Geometry check sheet. Reference: the model listing, model coordinates, mm. A direction names the side the tool comes from. Give positions to 0.01 mm unless a question says otherwise; leave off trailing zeros. Write each loop counter-clockwise with the first axis right and the second up, starting at its lowest first coordinate (ties: lowest second). Pieces come first, ordered by that corner, then holes. Notation, with made-up numbers: M 59,-38.75 L 94,-38.75 A14 cw 94,-19.75 Z; hole C -27,54 d4. An arc over 180 degrees is marked long. One line per item, written item: value. Start each with the question number.
1. Cross-section at C-C on y = 15. Record the cut outline in (x, z).
2. Cross-section at A-A on x = 21. Record the cut outline in (y, z).
3. Gauge pin test, flat ends, axial feed: pin 1 (2.5 mm diameter, centred on y = -16, z = 13.5, fed in from +X); pin 2 (4 mm diameter, centred on x = 22.5, z = 21, fed in from -Y); pin 3 (10.5 mm diameter, centred on y = 15, z = 14, fed in from -X). Record the tip position at first contact, or that the pin passes through.
4. Cross-section at B-B on z = 16.5. Record the cut outline in (x, y), then the cut area to 3 significant figures.
5. Release check for a two-part mould opening along Y. For faces 3 (the face through (0, 0, 24.5)), 4 (the face through (20, -15, 14)), 5 (the face through (-31.72, 1.4, 12.08)) record: pulls with the +Y half, pulls with the -Y half, needs draft (parallel to the pull), parting line crosses it, or undercut.
6. Tool access check on faces 1 (the face through (23.736, 11.034, 13.479)), 2 (the face through (0, 0, 0)). Record the directions out of +Z, -Z, +X, -X, +Y, -Y that give a thin tool (end or side, any length) a straight path to the whole face; none if there is none.
7. Cross-section at D-D on x = -14. Record the cut outline in (y, z).
8. Scan lines: line 1 (Y direction, x = 24.5, z = 14); line 2 (Y direction, x = 24.75, z = 14); line 3 (Z direction, x = 25.5, y = 15). Record each from-to range of solid material in increasing order.
from build123d import *

# Parameters (mm, degrees)
SKIZZE1_R        = 31.75
LIDAR_BASE_DEPTH = 24.5
SKIZZE2_R        = 4
SENSOR_CUT_DEPTH = 66.470413165


with BuildPart() as part:
    # Skizze1 → Lidar Base (new body)
    with BuildSketch(Plane.XY):
        Circle(SKIZZE1_R)
    extrude(amount=LIDAR_BASE_DEPTH)

    # Skizze2 → Sensor Cut (cut, through all)
    with BuildSketch(Plane(origin=(20, 0, 0), x_dir=(0, 0, -1), z_dir=(1, 0, 0))):
        with Locations(Location((-14, 15, 0), (0, 0, 180))):
            Circle(SKIZZE2_R)
        with Locations(Location((-14, -15, 0), (0, 0, 180))):
            Circle(SKIZZE2_R)
    extrude(amount=SENSOR_CUT_DEPTH, mode=Mode.SUBTRACT)


solid = part.part
Report:
1. outline: M -27.98,0 L 27.98,0 L 27.98,10 L 20,10 L 20,18 L 27.98,18 L 27.98,24.5 L -27.98,24.5 Z
2. outline: M -23.81,0 L 23.81,0 L 23.81,24.5 L -23.81,24.5 Z; hole C -15,14 d8; hole C 15,14 d8
3. pin 1: stops at x = 20
3. pin 2: stops at y = -24.24
3. pin 3: stops at x = -30.22
4. outline: M 20,-18.12 L 20,-11.88 L 29.44,-11.88 A31.75 ccw 29.44,11.88 L 20,11.88 L 20,18.12 L 26.07,18.12 A31.75 ccw long 26.07,-18.12 Z
4. area: 3,070 mm^2
5. face 3: needs draft
5. face 4: undercut
5. face 5: parting line crosses it
6. face 1: +X
6. face 2: -Z, +X, -X, +Y, -Y
7. outline: M -28.5,0 L 28.5,0 L 28.5,24.5 L -28.5,24.5 Z
8. line 1: y = -20.19 to -19, -11 to 11, 19 to 20.19
8. line 2: y = -19.89 to -19, -11 to 11, 19 to 19.89
8. line 3: z = 0 to 10, 18 to 24.5
